Build history of the part. All positions in model axes, mm. A direction names the side the tool comes from. Give positions to 0.01 mm unless a question says otherwise; leave off trailing zeros. Write each loop counter-clockwise with the first axis right and the second up, starting at its lowest first coordinate (ties: lowest second). Pieces come first, ordered by that corner, then holes. Notation, with made-up numbers: (76, -34.75) -> (129, -34.75) arc R10 ccw to (129, -18.75) -> close; hole circle Ø11 at (47.25, 75). An arc over 180 degrees is marked (long way). Put each result on its own line as item: value. Start each with the question number.
Item 1: Flat gauge pin, fed straight in: pin 1 Ø1.3 at (x, z) = (-2.5, 1.5) entering from +Y. Where does the tip first touch, or does it go through?
Item 2: Slice it at C-C, the plane x = 6. List the corners of the cut face in (y, z).
Item 3: Slice it at B-B, the plane y = -2.75. List the corners of the cut face in (x, z).
Item 4: Tool access for faces 5 (the flat face through (0, -7, 0)), 6 (the flat face through (3.482, 2.908, 1.282)): list every direction of +Z, -Z, +X, -X, +Y, -Y with a clear straight run to the whole face (end or side of a thin tool).
Item 5: Slice it at D-D, the plane x = 0. List the corners of the cut face in (y, z).
Item 6: Slice it at A-A, the plane z = 1.95. List the corners of the cut face in (x, y).
Item 7: Drill centre lines: line 1 along X through (y, z) = (-0.5, 1.55); line 2 along X through (y, z) = (2.5, 2.05); line 3 along Y through (x, z) = (-3.75, 2.4). Where is each one in solid material? Low to high.
Item 8: Two-plate mould, pull along X, no slides. Class faces 1 (the flat face through (11.025, -9, 1)), 2 (the flat face through (-11.025, -9, 1)), 3 (the flat face through (0, -11.3, 1)), 4 (the flat face through (0, -5.3, 1)): pulls with the +X half, pulls with the -X half, needs draft (parallel to the pull), parting line crosses it, or undercut.
```python
from build123d import *

# Parameters (mm, degrees)
BOSS_EXTRUDE1_DEPTH = 2.6
SKETCH2_W           = 22.04953915
SKETCH2_H           = 2.6
BOSS_EXTRUDE2_DEPTH = 4


with BuildPart() as part:
    # Sketch1 → Boss-Extrude1 (new body)
    with BuildSketch(Plane.XY):
        Polygon((4.274769575, 3.5), (2.666274292, 2.3), (5.254399491, -1.841000318), (7.416274292, -5.3), (-7.416274292, -5.3), (-5.254399491, -1.841000318), (-2.754399491, 2.158999682), (-4.274769575, 3.5), (-6.950396099, -0.781002438), (-11.024769575, -7.3), (11.024769575, -7.3), (6.950396099, -0.781002438), align=None)
    extrude(amount=BOSS_EXTRUDE1_DEPTH)

    # Sketch2 → Boss-Extrude2 (add)
    with BuildSketch(Plane.XZ.offset(7.3)):
        with Locations((0, 1.3)):
            Rectangle(SKETCH2_W, SKETCH2_H)
    extrude(amount=BOSS_EXTRUDE2_DEPTH)


solid = part.part
```
Values follow:
1. pin 1: y = 2.51
2. outline: (-11.3, 0) -> (-5.3, 0) -> (-5.3, 2.6) -> (-11.3, 2.6) -> close; (-3.03, 0) -> (0.74, 0) -> (0.74, 2.6) -> (-3.03, 2.6) -> close
3. outline: (-8.18, 0) -> (-5.82, 0) -> (-5.82, 2.6) -> (-8.18, 2.6) -> close; (5.82, 0) -> (8.18, 0) -> (8.18, 2.6) -> (5.82, 2.6) -> close
4. face 5: -Z, +X, -X, +Y, -Y
4. face 6: +Z, -Z, +Y
5. outline: (-11.3, 0) -> (-5.3, 0) -> (-5.3, 2.6) -> (-11.3, 2.6) -> close
6. outline: (-11.02, -11.3) -> (11.02, -11.3) -> (11.02, -7.3) -> (4.27, 3.5) -> (2.67, 2.3) -> (7.42, -5.3) -> (-7.42, -5.3) -> (-2.75, 2.16) -> (-4.27, 3.5) -> (-11.02, -7.3) -> close
7. line 1: -6.77 to -4.42, 4.42 to 6.77
7. line 2: -4.9 to -3.14, 2.93 to 4.9
7. line 3: -11.3 to -5.3, 0.57 to 3.04
8. face 1: pulls with the +X half
8. face 2: pulls with the -X half
8. face 3: needs draft
8. face 4: undercut
